Source: CAD feature listing. Evaluate the final solid. Frame: model axes, mm. A direction names the side the tool comes from. Give positions to 0.01 mm unless a question says otherwise; leave off trailing zeros. Loops run counter-clockwise (first coordinate to the right, second up) from the corner with the lowest first, then second, coordinate; pieces in that order, holes last. Notation, with made-up numbers: (67, -33) -> (100, -33) arc R15 ccw to (100, -26) -> close; hole circle Ø2 at (16, 84). An arc over 180 degrees is marked (long way). Put each result on its own line as item: value.
```python
from build123d import *

# Parameters (mm, degrees)
SKETCH1_W           = 76.2
SKETCH1_H           = 127
BOSS_EXTRUDE1_DEPTH = 12.7
SKETCH2_W           = 76.2
SKETCH2_H           = 38.1
BOSS_EXTRUDE2_DEPTH = 12.7
SKETCH3_R           = 9.525
CUT_EXTRUDE1_DEPTH  = 149.649688866
FILLET1_R           = 25.4
CHAMFER1_SIZE       = 3.175
SHELL1_T            = -2.54


with BuildPart() as part:
    # Sketch1 → Boss-Extrude1 (new body)
    with BuildSketch(Plane.XY):
        with Locations((-38.1, -63.5)):
            Rectangle(SKETCH1_W, SKETCH1_H)
    extrude(amount=BOSS_EXTRUDE1_DEPTH)

    # Sketch2 → Boss-Extrude2 (add)
    with BuildSketch(Plane.XY.offset(12.7)):
        with Locations((-38.1, -107.95)):
            Rectangle(SKETCH2_W, SKETCH2_H)
    extrude(amount=BOSS_EXTRUDE2_DEPTH)

    # Sketch3 → Cut-Extrude1 (cut, through all)
    with BuildSketch(Plane.XY.offset(12.7)):
        with Locations((-50.8, -25.4)):
            Circle(SKETCH3_R)
    extrude(amount=-CUT_EXTRUDE1_DEPTH, mode=Mode.SUBTRACT)

    # Fillet1
    fillet1_edges = [part.edges().sort_by_distance(p)[0] for p in [
        (0, -88.9, 19.05),
        (0, 0, 6.35),
    ]]
    fillet(fillet1_edges, radius=FILLET1_R)

    # Chamfer1
    chamfer1_edges = [part.edges().sort_by_distance(p)[0] for p in [
        (0, -69.85, 12.7),
        (0, -120.65, 25.4),
        (-50.8, -88.9, 25.4),
        (-7.439487758, -96.339487758, 25.4),
        (-50.8, 0, 12.7),
        (-7.439487758, -7.439487758, 12.7),
    ]]
    chamfer(chamfer1_edges, length=CHAMFER1_SIZE)

    # Shell1
    shell1_openings = [part.faces().sort_by_distance(p)[0] for p in [
        (-60.325, -25.4, 6.35),
        (-38.193985292, -65.538658625, 0),
        (-38.196714534, -127, 12.669604003),
        (-76.2, -73.894162641, 9.238687601),
    ]]
    offset(amount=SHELL1_T, openings=shell1_openings, kind=Kind.INTERSECTION)


solid = part.part
```
(1) First-contact query: P1, Ø10, axis at x = -47.5, y = -69.5, coming from the +Z side; P2, Ø5, axis at x = -37, z = 20, coming from the -Y side; P3, Ø9, axis at x = -46, z = 16.5, coming from the -Y side. Flat tips, straight axial feed; report the tip coordinate or a pass-through.
Calculated:
P1: stops at z = 12.7
P2: stops at y = -92.77
P3: stops at y = -91.44
(2) Section C-C on y = -65. Return loops of the section in (x, z) (3 decimals), then the cut area to 3 significant figures.
Calculated:
outline: (-76.2, 10.16) -> (-4.227, 10.16) -> (-2.54, 8.473) -> (-2.54, 0) -> (0, 0) -> (0, 9.525) -> (-3.175, 12.7) -> (-76.2, 12.7) -> close
area: 216 mm²
(3) Reachability of faces 4 (the flat face through (-76.2, -64, 12)), 5 (the flat face through (-1.565, -69.228, 11.09)), 6 (the flat face through (-41, -110, 22.86)) from +Z, -Z, +X, -X, +Y, -Y: full face, straight path, thin tool, end or side. Return the list, or none.
Calculated:
face 4: +Z, -Z, -X, +Y, -Y
face 5: +Z, +X, +Y
face 6: -Z, -X, -Y
(4) Section D-D on z = 3.5. Return loops of the section in (x, y), then the cut area to 3 significant figures.
Calculated:
outline: (-76.2, -2.54) -> (-25.4, -2.54) arc R22.86 cw to (-2.54, -25.4) -> (-2.54, -127) -> (0, -127) -> (0, -25.4) arc R25.4 ccw to (-25.4, 0) -> (-76.2, 0) -> close
area: 483 mm²
(5) Section B-B on y = -30. Return loops of the section in (x, z) (3 decimals).
Calculated:
outline: (-76.2, 10.16) -> (-59.141, 10.16) -> (-59.141, 12.7) -> (-76.2, 12.7) -> close; (-42.459, 10.16) -> (-4.227, 10.16) -> (-2.54, 8.473) -> (-2.54, 0) -> (0, 0) -> (0, 9.525) -> (-3.175, 12.7) -> (-42.459, 12.7) -> close
(6) Draft query along X for faces 1 (the flat face through (-51, -91.44, 16)), 2 (the conical face through (-9.12, -98.37, 24.85)), 3 (the cylindrical face through (-45.68, -17.37, 11.45)). Return one class per face: released by +X, released by -X, zero draft, split by the parting line, or undercut.
Calculated:
face 1: zero draft
face 2: released by +X
face 3: undercut
(7) Line query: probe 1 along Z at (x, y) = (-57, -100); probe 2 along Y at (x, z) = (-36, 3.75); probe 3 along Z at (x, y) = (-34.5, -65.5). Output: solid intervals per line, ascending. Write a range as from..to.
Calculated:
probe 1: z = 22.86..25.4
probe 2: y = -2.54..0
probe 3: z = 10.16..12.7
(8) Section A-A on x = -50.8. Return loops of the section in (y, z) (3 decimals).
Calculated:
outline: (-127, 22.86) -> (-93.127, 22.86) -> (-91.44, 21.173) -> (-91.44, 10.16) -> (-34.925, 10.16) -> (-34.925, 12.7) -> (-88.9, 12.7) -> (-88.9, 22.225) -> (-92.075, 25.4) -> (-127, 25.4) -> close; (-15.875, 10.16) -> (-4.227, 10.16) -> (-2.54, 8.473) -> (-2.54, 0) -> (0, 0) -> (0, 9.525) -> (-3.175, 12.7) -> (-15.875, 12.7) -> close
